Design review of the part built by this model. Coordinates are the model's own, in mm. Face numbers are marked on the shaded views. A direction names the side the tool comes from. Coordinates: 2 decimals unless noted, no trailing zeros. Order: outer loops, then holes, each group sorted by start corner. A loop starts at its lowest first (then second) coordinate and runs counter-clockwise, first axis right, second up. Notation, with made-up numbers: (6.5, 33) -> (44.5, 33) arc R30 ccw to (44.5, 55) -> close; hole circle Ø9 at (49.25, 57). An arc over 180 degrees is marked (long way). Use a Markdown table: item, result. Add a question column.
Q1. Add section A-A (z = 32.5). State the section outline as (x, y) points.
Q2. Add section B-B (y = 7.5). State the section outline as (x, z) points.
Q3. Insertion check: pin 1 (2 mm diameter, centred on y = -13, z = 42, fed in from -X). The pin has a flat end and moves straight along its axis. Give the tip position at first contact, or say it passes through.
Q4. Wall thickness on probe 1 along X at (y, z) = (-9.5, 45); probe 2 along Y at (x, z) = (2.5, 31); probe 3 along Y at (x, z) = (5.25, 16): over which ranges is each line inside the solid? List them lowest first.
Q5. Machinability: for the marked faces 1 and 2, which of the approach directions +Z, -Z, +X, -X, +Y, -Y give a long, thin tool a straight path to every point of the face, cutting with its end or side? Answer none if there is none.
Q6. Add section C-C (x = -1.25). State the section outline as (y, z) points, then the cut area to 3 significant figures.
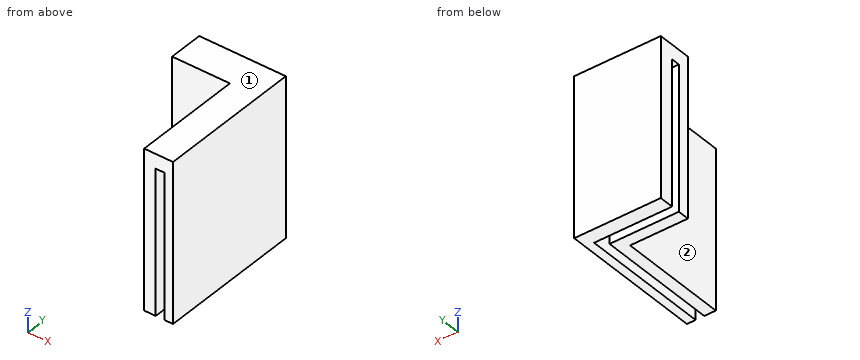
from build123d import *

# Parameters (mm, degrees)
BOSS_EXTRUDE1_DEPTH   = 55
BOSS_EXTRUDE1_2_DEPTH = 55
SKETCH2_W             = 4
SKETCH2_H             = 38
SKETCH2_W_2           = 6
BOSS_EXTRUDE2_DEPTH   = 5


with BuildPart() as part:
    # Sketch1 → Boss-Extrude1 (new body)
    with BuildSketch(Plane.XY):
        Polygon((9, 17), (-15, 17), (-15, 13), (5, 13), (5, -25), (9, -25), align=None)
    extrude(amount=BOSS_EXTRUDE1_DEPTH)



with BuildPart() as body_2:
    # Sketch1 → Boss-Extrude1 2 (new body)
    with BuildSketch(Plane.XY):
        Polygon((-15, 25), (-15, 20), (12, 20), (12, -25), (15, -25), (15, 25), align=None)
    extrude(amount=BOSS_EXTRUDE1_2_DEPTH)


with BuildPart() as part_1:
    add(part.part)

    add(body_2.part)  # Boss-Extrude2 merges body 2
    # Sketch2 → Boss-Extrude2 (add)
    with BuildSketch(Plane.XY.offset(55)):
        Polygon((-15, 25), (-15, 17), (9, 17), (9, 13), (15, 13), (15, 25), align=None)
        Polygon((-15, 17), (-15, 13), (5, 13), (9, 13), (9, 17), align=None)
        with Locations((7, -6)):
            Rectangle(SKETCH2_W, SKETCH2_H)
        with Locations((12, -6)):
            Rectangle(SKETCH2_W_2, SKETCH2_H)
    extrude(amount=-BOSS_EXTRUDE2_DEPTH)


solid = part_1.part
Established:
| question | item | result |
|---|---|---|
| 1 | outline | (-15, 13) -> (5, 13) -> (5, -25) -> (9, -25) -> (9, 17) -> (-15, 17) -> close; (-15, 20) -> (12, 20) -> (12, -25) -> (15, -25) -> (15, 25) -> (-15, 25) -> close |
| 2 | outline | (5, 0) -> (9, 0) -> (9, 50) -> (12, 50) -> (12, 0) -> (15, 0) -> (15, 55) -> (5, 55) -> close |
| 3 | pin 1 | x = 5 |
| 4 | probe 1 | 5 to 9, 12 to 15 |
| 4 | probe 2 | 13 to 17, 20 to 25 |
| 4 | probe 3 | -25 to 17, 20 to 25 |
| 5 | face 1 | +Z, +X, -X, +Y, -Y |
| 5 | face 2 | +Z, -Z, -X, -Y |
| 6 | outline | (13, 0) -> (17, 0) -> (17, 50) -> (20, 50) -> (20, 0) -> (25, 0) -> (25, 55) -> (13, 55) -> close |
| 6 | area | 510 mm^2 |
